Source: CAD feature listing. Evaluate the final solid. Frame: model axes, mm. Round coordinates to 2 decimals unless told otherwise and drop trailing zeros. Order: outer loops, then holes, each group sorted by start corner. A loop starts at its lowest first (then second) coordinate and runs counter-clockwise, first axis right, second up. Notation, with made-up numbers: M -12,-5.5 L -8,-5.5 A19 cw -8,10.5 Z; hole C -10.75,-8.75 d4. An arc over 180 degrees is marked long. Use CSV: the item, a comma, the result in double quotes. Start each with the question number.
```python
from build123d import *

# Parameters (mm, degrees)
SKETCH1_R           = 7
SKETCH1_R_2         = 2.025
SKETCH1_R_3         = 2.05
BOSS_EXTRUDE1_DEPTH = 3.15
CUT_EXTRUDE1_DEPTH  = 3.15
BOSS_EXTRUDE2_START = -3.15
SKETCH3_R           = 2
SKETCH3_R_2         = 7
SKETCH3_R_3         = 2.025
SKETCH3_R_4         = 11
BOSS_EXTRUDE2_DEPTH = 3.15


with BuildPart() as part:
    # Sketch1 → Boss-Extrude1 (new body)
    with BuildSketch(Plane(origin=(0, 0, 0), x_dir=(1, 0, 0), z_dir=(0, 1, 0))):
        with BuildLine():
            Line((51.028117024, 31.392984288), (48.107015586, 31.392984288))
            ThreePointArc((48.107015586, 31.392984288), (44.57148168, 29.928518194), (43.107015586, 26.392984288))
            Line((43.107015586, 26.392984288), (43.107015586, 8.3528051))
            ThreePointArc((43.107015586, 8.3528051), (35.212895347, -7.567234951), (17.762248065, -10.919803965))
            Line((17.762248065, -10.919803965), (-6.126047208, -4.29499337))
            ThreePointArc((-6.126047208, -4.29499337), (-21.319285931, -6.160488515), (-30.743423793, -18.222834912))
            ThreePointArc((-30.743423793, -18.222834912), (-28.877928648, -33.416073636), (-16.815582251, -42.840211498))
            Line((-16.815582251, -42.840211498), (26.065972917, -54.732319234))
            ThreePointArc((26.065972917, -54.732319234), (41.259211641, -52.866824088), (50.683349503, -40.804477691))
            Line((50.683349503, -40.804477691), (56.028117024, -21.531868627))
            Line((56.028117024, -21.531868627), (56.028117024, 26.392984288))
            ThreePointArc((56.028117024, 26.392984288), (54.56365093, 29.928518194), (51.028117024, 31.392984288))
        make_face()
        with Locations(Location((35.265262251, -36.528663674, 0), (0, 0, 270))):
            Circle(SKETCH1_R, mode=Mode.SUBTRACT)
        with Locations(Location((-15.325336542, -22.49864893, 0), (0, 0, 270))):
            Circle(SKETCH1_R, mode=Mode.SUBTRACT)
        with Locations(Location((-5.478385908, -16.927512313, 0), (0, 0, 270))):
            Circle(SKETCH1_R_2, mode=Mode.SUBTRACT)
        with Locations(Location((-9.754199925, -32.345599564, 0), (0, 0, 270))):
            Circle(SKETCH1_R_2, mode=Mode.SUBTRACT)
        with Locations(Location((-25.172287176, -28.069785547, 0), (0, 0, 270))):
            Circle(SKETCH1_R_2, mode=Mode.SUBTRACT)
        with Locations(Location((-20.896473159, -12.651698295, 0), (0, 0, 270))):
            Circle(SKETCH1_R_2, mode=Mode.SUBTRACT)
        with Locations(Location((-13.725837034, -7.376096191, 0), (0, 0, 270))):
            Circle(SKETCH1_R_2, mode=Mode.SUBTRACT)
        with Locations(Location((49.567566305, 24.392984288, 0), (0, 0, 270))):
            Circle(SKETCH1_R_3, mode=Mode.SUBTRACT)
    extrude(amount=BOSS_EXTRUDE1_DEPTH)

    # Sketch2 → Cut-Extrude1 (cut)
    with BuildSketch(Plane(origin=(0, 3.15, 0), x_dir=(1, 0, 0), z_dir=(0, 1, 0))):
        Polygon((0, 8.660254038), (-7.5, 4.330127019), (-7.5, -4.330127019), (0, -8.660254038), (7.5, -4.330127019), (7.5, 4.330127019), align=None)
        Polygon((21, 8.660254038), (13.5, 4.330127019), (13.5, -4.330127019), (21, -8.660254038), (28.5, -4.330127019), (28.5, 4.330127019), align=None)
        Polygon((10.5, -9.526279442), (3, -13.856406461), (3, -22.516660498), (10.5, -26.846787517), (18, -22.516660498), (18, -13.856406461), align=None)
        Polygon((31.5, -9.526279442), (24, -13.856406461), (24, -22.516660498), (31.5, -26.846787517), (39, -22.516660498), (39, -13.856406461), align=None)
        Polygon((52.5, -9.526279442), (45, -13.856406461), (45, -22.516660498), (52.5, -26.846787517), (60, -22.516660498), (60, -13.856406461), align=None)
        Polygon((42, 8.660254038), (34.5, 4.330127019), (34.5, -4.330127019), (42, -8.660254038), (49.5, -4.330127019), (49.5, 4.330127019), align=None)
        Polygon((63, 8.660254038), (55.5, 4.330127019), (55.5, -4.330127019), (63, -8.660254038), (70.5, -4.330127019), (70.5, 4.330127019), align=None)
        Polygon((73.5, -9.526279442), (66, -13.856406461), (66, -22.516660498), (73.5, -26.846787517), (81, -22.516660498), (81, -13.856406461), align=None)
        Polygon((52.5, -45.899346401), (45, -50.229473419), (45, -58.889727457), (52.5, -63.219854476), (60, -58.889727457), (60, -50.229473419), align=None)
        Polygon((42, -27.712812921), (34.5, -32.04293994), (34.5, -40.703193978), (42, -45.033320997), (49.5, -40.703193978), (49.5, -32.04293994), align=None)
        Polygon((63, -27.712812921), (55.5, -32.04293994), (55.5, -40.703193978), (63, -45.033320997), (70.5, -40.703193978), (70.5, -32.04293994), align=None)
        Polygon((73.5, -45.899346401), (66, -50.229473419), (66, -58.889727457), (73.5, -63.219854476), (81, -58.889727457), (81, -50.229473419), align=None)
        Polygon((10.5, -45.899346401), (3, -50.229473419), (3, -58.889727457), (10.5, -63.219854476), (18, -58.889727457), (18, -50.229473419), align=None)
        Polygon((0, -27.712812921), (-7.5, -32.04293994), (-7.5, -40.703193978), (0, -45.033320997), (7.5, -40.703193978), (7.5, -32.04293994), align=None)
        Polygon((21, -27.712812921), (13.5, -32.04293994), (13.5, -40.703193978), (21, -45.033320997), (28.5, -40.703193978), (28.5, -32.04293994), align=None)
        Polygon((31.5, -45.899346401), (24, -50.229473419), (24, -58.889727457), (31.5, -63.219854476), (39, -58.889727457), (39, -50.229473419), align=None)
        Polygon((-21, -27.712812921), (-28.5, -32.04293994), (-28.5, -40.703193978), (-21, -45.033320997), (-13.5, -40.703193978), (-13.5, -32.04293994), align=None)
        Polygon((-10.5, -9.526279442), (-18, -13.856406461), (-18, -22.516660498), (-10.5, -26.846787517), (-3, -22.516660498), (-3, -13.856406461), align=None)
        Polygon((-21, 8.660254038), (-28.5, 4.330127019), (-28.5, -4.330127019), (-21, -8.660254038), (-13.5, -4.330127019), (-13.5, 4.330127019), align=None)
        Polygon((-10.5, -45.899346401), (-18, -50.229473419), (-18, -58.889727457), (-10.5, -63.219854476), (-3, -58.889727457), (-3, -50.229473419), align=None)
        Polygon((-42, -27.712812921), (-49.5, -32.04293994), (-49.5, -40.703193978), (-42, -45.033320997), (-34.5, -40.703193978), (-34.5, -32.04293994), align=None)
        Polygon((-31.5, -9.526279442), (-39, -13.856406461), (-39, -22.516660498), (-31.5, -26.846787517), (-24, -22.516660498), (-24, -13.856406461), align=None)
        Polygon((-42, 8.660254038), (-49.5, 4.330127019), (-49.5, -4.330127019), (-42, -8.660254038), (-34.5, -4.330127019), (-34.5, 4.330127019), align=None)
        Polygon((-31.5, -45.899346401), (-39, -50.229473419), (-39, -58.889727457), (-31.5, -63.219854476), (-24, -58.889727457), (-24, -50.229473419), align=None)
        Polygon((42, 45.033320997), (34.5, 40.703193978), (34.5, 32.04293994), (42, 27.712812921), (49.5, 32.04293994), (49.5, 40.703193978), align=None)
        Polygon((63, 45.033320997), (55.5, 40.703193978), (55.5, 32.04293994), (63, 27.712812921), (70.5, 32.04293994), (70.5, 40.703193978), align=None)
        Polygon((73.5, 26.846787517), (66, 22.516660498), (66, 13.856406461), (73.5, 9.526279442), (81, 13.856406461), (81, 22.516660498), align=None)
        Polygon((52.5, 26.846787517), (45, 22.516660498), (45, 13.856406461), (52.5, 9.526279442), (60, 13.856406461), (60, 22.516660498), align=None)
    extrude(amount=-CUT_EXTRUDE1_DEPTH, mode=Mode.SUBTRACT)

    # Sketch3 → Boss-Extrude2 (add)
    # profile 1 of 2: a face of its own
    with BuildSketch(Plane(origin=(0, 3.15, 0), x_dir=(1, 0, 0), z_dir=(0, 1, 0)).offset(BOSS_EXTRUDE2_START)):
        with BuildLine():
            Line((50.793806272, 31.392984288), (48.107015586, 31.392984288))
            ThreePointArc((48.107015586, 31.392984288), (44.57148168, 29.928518194), (43.107015586, 26.392984288))
            Line((43.107015586, 26.392984288), (43.107015586, 8.3528051))
            ThreePointArc((43.107015586, 8.3528051), (35.212895347, -7.567234951), (17.762248065, -10.919803965))
            Line((17.762248065, -10.919803965), (-6.126047208, -4.29499337))
            ThreePointArc((-6.126047208, -4.29499337), (-20.562647206, -5.753602821), (-30.213693877, -16.588742838))
            ThreePointArc((-30.213693877, -16.588742838), (-29.284814342, -32.659434911), (-16.815582251, -42.840211498))
            Line((-16.815582251, -42.840211498), (26.065972917, -54.732319234))
            ThreePointArc((26.065972917, -54.732319234), (41.259211641, -52.866824088), (50.683349503, -40.804477691))
            Line((50.683349503, -40.804477691), (56.028117024, -21.531868627))
            Line((56.028117024, -21.531868627), (56.028117024, 27.690214825))
            ThreePointArc((56.028117024, 27.690214825), (54.073099239, 30.477610817), (50.793806272, 31.392984288))
        make_face()
        with Locations(Location((49.567566305, 24.392984288, 0), (0, 0, 270))):
            Circle(SKETCH3_R, mode=Mode.SUBTRACT)
        with Locations(Location((-15.325336542, -22.49864893, 0), (0, 0, 270))):
            Circle(SKETCH3_R_2, mode=Mode.SUBTRACT)
        with Locations(Location((-20.896473159, -12.651698295, 0), (0, 0, 270))):
            Circle(SKETCH3_R_3, mode=Mode.SUBTRACT)
        with Locations(Location((-13.725837034, -7.376096191, 0), (0, 0, 270))):
            Circle(SKETCH3_R_3, mode=Mode.SUBTRACT)
        with Locations(Location((-25.172287176, -28.069785547, 0), (0, 0, 270))):
            Circle(SKETCH3_R_3, mode=Mode.SUBTRACT)
        with Locations(Location((-9.754199925, -32.345599564, 0), (0, 0, 270))):
            Circle(SKETCH3_R_3, mode=Mode.SUBTRACT)
        with Locations(Location((-5.478385908, -16.927512313, 0), (0, 0, 270))):
            Circle(SKETCH3_R_3, mode=Mode.SUBTRACT)
        with BuildLine():
            Line((47.107015586, 21.239305458), (47.107015586, 8.3528051))
            ThreePointArc((47.107015586, 8.3528051), (37.634071299, -10.751242961), (16.69329456, -14.774325777))
            Line((16.69329456, -14.774325777), (-7.195000712, -8.149515183))
            ThreePointArc((-7.195000712, -8.149515183), (-8.443375133, -7.856631443), (-9.711193989, -7.66465507))
            ThreePointArc((-9.711193989, -7.66465507), (-13.17062628, -11.36261924), (-17.508855114, -8.750650375))
            ThreePointArc((-17.508855114, -8.750650375), (-18.103373072, -9.007067766), (-18.687030177, -9.287328115))
            ThreePointArc((-18.687030177, -9.287328115), (-17.142141715, -11.200622691), (-16.998671761, -13.655575412))
            ThreePointArc((-16.998671761, -13.655575412), (-12.920191157, -13.825974851), (-9.336488748, -15.780486823))
            ThreePointArc((-9.336488748, -15.780486823), (-1.975204232, -14.945507483), (-6.482263024, -20.82531371))
            ThreePointArc((-6.482263024, -20.82531371), (-6.652662463, -24.903794314), (-8.607174435, -28.487496724))
            ThreePointArc((-8.607174435, -28.487496724), (-7.772195096, -35.84878124), (-13.652001323, -31.341722448))
            ThreePointArc((-13.652001323, -31.341722448), (-17.730481927, -31.171323009), (-21.314184336, -29.216811037))
            ThreePointArc((-21.314184336, -29.216811037), (-22.701556213, -31.247223745), (-25.01120364, -32.091560913))
            ThreePointArc((-25.01120364, -32.091560913), (-21.022595954, -36.403625004), (-15.746628746, -38.985689685))
            Line((-15.746628746, -38.985689685), (27.134926421, -50.877797421))
            ThreePointArc((27.134926421, -50.877797421), (39.2895174, -49.385401305), (46.82882769, -39.735524187))
            Line((46.82882769, -39.735524187), (52.028117024, -20.987492519))
            Line((52.028117024, -20.987492519), (52.028117024, 21.239305458))
            ThreePointArc((52.028117024, 21.239305458), (49.567566305, 20.392984288), (47.107015586, 21.239305458))
        make_face(mode=Mode.SUBTRACT)
        with BuildLine():
            ThreePointArc((-26.465118047, -17.984514757), (-27.31052728, -21.308508299), (-27.428073888, -24.736311186))
            ThreePointArc((-27.428073888, -24.736311186), (-25.8588989, -24.103781344), (-24.16841006, -24.171984149))
            ThreePointArc((-24.16841006, -24.171984149), (-23.998010621, -20.093503545), (-22.043498649, -16.509801136))
            ThreePointArc((-22.043498649, -16.509801136), (-23.527657447, -15.697596232), (-24.546925983, -14.34722747))
            ThreePointArc((-24.546925983, -14.34722747), (-25.623358962, -16.103991261), (-26.465118047, -17.984514757))
        make_face(mode=Mode.SUBTRACT)
    # profile 2 of 2: a face of its own
    with BuildSketch(Plane(origin=(0, 3.15, 0), x_dir=(1, 0, 0), z_dir=(0, 1, 0)).offset(BOSS_EXTRUDE2_START)):
        with Locations((35.265262251, -36.528663674)):
            Circle(SKETCH3_R_4)
        with Locations(Location((35.265262251, -36.528663674, 0), (0, 0, 270))):
            Circle(SKETCH3_R_2, mode=Mode.SUBTRACT)
    extrude(amount=BOSS_EXTRUDE2_DEPTH)


solid = part.part
```
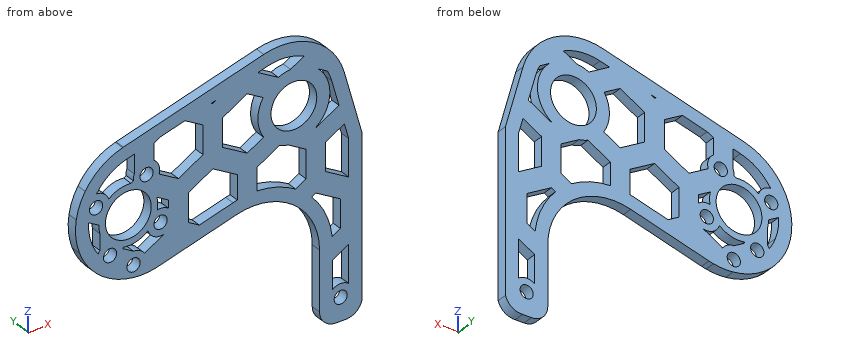
(1) Section C-C on y = 0.6. Give the number of separate pieces and of enclosed holes in the cut face, plus the area to 3 significant figures.
(2) Section B-B on x = 22. Return loops of the section in (y, z), plus the area to 3 significant figures.
(3) Contact query for flat-ended pins moving along their axis: P1, Ø0.9, axis at y = 1, z = 37.5, coming from the +X side; P2, Ø1, axis at x = 34, y = 2, coming from the +Z side; P3, Ø1.3, axis at x = 49.5, y = 1, coming from the -Z side. Output: stop coordinate, or through.
(4) Section A-A on z = -24. Return loops of the section in (x, y), plus the area to 3 significant figures.
(5) Line query: line 1 along X through (y, z) = (2.5, -15.5); line 2 along Z through (x, y) = (5.5, 0.4); line 3 along Z through (x, y) = (-21, 0.5). Output: solid intervals per line, ascending.
Results below:
1,separate pieces,"1"
1,enclosed holes,"22"
1,area,"2,500 mm2"
2,outline,"M 0,11.62 L 3.15,11.62 L 3.15,28.29 L 0,28.29 Z; M 0,44.46 L 3.15,44.46 L 3.15,53.6 L 0,53.6 Z"
2,area,"81.3 mm2"
3,P1,"stops at x = 51.72"
3,P2,"stops at z = 55.35"
3,P3,"stops at z = -31.39"
4,outline,"M 43.11,0 L 47.61,0 L 47.61,3.15 L 43.11,3.15 Z; M 51.53,0 L 56.03,0 L 56.03,3.15 L 51.53,3.15 Z"
4,area,"28.3 mm2"
5,line 1,"x = 43.11 to 47.11, 52.03 to 56.03"
5,line 2,"z = 7.52 to 12.41, 23.96 to 30.89, 41.86 to 49.03"
5,line 3,"z = 5.98 to 10.63, 14.67 to 18.4, 26.6 to 29.48, 36.42 to 41.15"
